from build123d import *

# Parameters (mm, degrees)
EXTRUDE_1_DEPTH                 = 52
CUT_EXTRUDE_1_REACH             = 161.013
CUT_EXTRUDE_1_DIRECTION_2_DEPTH = 7
SKETCH_3_R                      = 1.5
SKETCH_3_R_2                    = 3
CUT_EXTRUDE_2_DEPTH             = 160.138304628
FILLET_1_R                      = 5
CHAMFER_1_SIZE                  = 5
FILLET_2_R                      = 12.5
EXTRUDE_2_DEPTH                 = 9
EXTRUDE_3_DEPTH                 = 9
EXTRUDE_3_DEPTH_BACK            = 2
CHAMFER_3_SIZE                  = 6
EXTRUDE_START                   = -11
SKETCH_7_R                      = 1.6
EXTRUDE_4_DEPTH                 = 2


with BuildPart() as part:
    # 草图1 → 凸台-拉伸1 (new body)
    with BuildSketch(Plane(origin=(0, 0, 0), x_dir=(0, 0, -1), z_dir=(1, 0, 0))):
        Polygon((0, 0), (0, 98), (-9, 98), (-9, 150), (-7, 150), (-7, 100), (2, 100), (2, 0), align=None)
    extrude(amount=EXTRUDE_1_DEPTH)

    # 草图2 → 切除-拉伸1 (cut, up to next)
    with BuildSketch(Plane(origin=(0, 0, 7), x_dir=(-1, 0, 0), z_dir=(0, 0, -1)), mode=Mode.PRIVATE) as cut_extrude_1_sk1:
        Polygon((-49, 146), (-49, 123), (-24, 123), (-24, 128.5), (-14, 128.5), (-14, 117), (-41, 117), (-41, 106), (-31, 106), (-31, 98), (-17, 98), (-17, 106), (-4, 106), (-4, 140.5), (-24, 140.5), (-24, 146), align=None)
    cut_extrude_1_tool1 = extrude(cut_extrude_1_sk1.sketch, amount=-CUT_EXTRUDE_1_REACH, mode=Mode.PRIVATE) & part.part
    add(cut_extrude_1_tool1.solids().sort_by_distance((25.692202, 124.595066, 7))[0], mode=Mode.SUBTRACT)

    # 草图2 → 切除-拉伸1 direction 2 (cut)
    with BuildSketch(Plane(origin=(0, 0, 7), x_dir=(-1, 0, 0), z_dir=(0, 0, -1))):
        Polygon((-49, 146), (-49, 123), (-24, 123), (-24, 128.5), (-14, 128.5), (-14, 117), (-41, 117), (-41, 106), (-31, 106), (-31, 98), (-17, 98), (-17, 106), (-4, 106), (-4, 140.5), (-24, 140.5), (-24, 146), align=None)
    extrude(amount=CUT_EXTRUDE_1_DIRECTION_2_DEPTH, mode=Mode.SUBTRACT)

    # 草图3 → 切除-拉伸2 (cut, through all)
    with BuildSketch(Plane(origin=(0, 0, -2), x_dir=(-1, 0, 0), z_dir=(0, 0, -1))):
        with Locations(Location((-15.5, 19, 0), (0, 0, 90))):
            Circle(SKETCH_3_R)
        with Locations(Location((-12, 19, 0), (0, 0, 90))):
            Circle(SKETCH_3_R)
        with Locations(Location((-8.5, 19, 0), (0, 0, 90))):
            Circle(SKETCH_3_R)
        with Locations(Location((-8.5, 5, 0), (0, 0, 90))):
            Circle(SKETCH_3_R)
        with Locations(Location((-12, 5, 0), (0, 0, 90))):
            Circle(SKETCH_3_R)
        with Locations(Location((-15.5, 5, 0), (0, 0, 90))):
            Circle(SKETCH_3_R)
        with Locations(Location((-5, 15.5, 0), (0, 0, 90))):
            Circle(SKETCH_3_R)
        with Locations(Location((-5, 12, 0), (0, 0, 90))):
            Circle(SKETCH_3_R)
        with Locations(Location((-5, 8.5, 0), (0, 0, 90))):
            Circle(SKETCH_3_R)
        with Locations(Location((-19, 8.5, 0), (0, 0, 90))):
            Circle(SKETCH_3_R)
        with Locations(Location((-19, 12, 0), (0, 0, 90))):
            Circle(SKETCH_3_R)
        with Locations(Location((-19, 15.5, 0), (0, 0, 90))):
            Circle(SKETCH_3_R)
        with Locations(Location((-8, 145, 0), (0, 0, 90))):
            Circle(SKETCH_3_R)
        with Locations(Location((-47, 116, 0), (0, 0, 90))):
            Circle(SKETCH_3_R)
        with Locations(Location((-18, 145, 0), (0, 0, 90))):
            Circle(SKETCH_3_R)
        with Locations(Location((-12, 12, 0), (0, 0, 90))):
            Circle(SKETCH_3_R_2)
        Polygon((-42, 75), (-22, 0), (-52, 0), (-52, 115), (-42, 100), align=None)
        with BuildLine():
            Line((0, 100), (-10.111173925, 100))
            ThreePointArc((-10.111173925, 100), (-23.988643866, 58.568340451), (0, 22.048324701))
            Line((0, 22.048324701), (0, 100))
        make_face()
    extrude(amount=-CUT_EXTRUDE_2_DEPTH, mode=Mode.SUBTRACT)

    # 圆角1
    fillet_1_edges = [part.edges().sort_by_distance(p)[0] for p in [
        (0, 100, 8),
        (52, 115, 8),
        (52, 150, 8),
        (14, 128.5, 8),
        (14, 117, 8),
        (4, 106, 8),
        (4, 140.5, 8),
        (0, 150, 8),
    ]]
    fillet(fillet_1_edges, radius=FILLET_1_R)

    # 倒角1
    chamfer_1_edges = [part.edges().sort_by_distance(p)[0] for p in [
        (36.5, 100, 7),
        (13.555586963, 100, 7),
    ]]
    chamfer(chamfer_1_edges, length=CHAMFER_1_SIZE)

    # 圆角2
    # the kernel refuses this fillet: 12.5 mm, written as the material it takes off along each edge
    with BuildSketch(Plane(origin=(22, 0, -26.008697284), x_dir=(0.2576626505603326, 0.9662349396012463, 0), z_dir=(0, 0, 1))) as fillet_2_piece_1:
        with BuildLine():
            CenterArc((FILLET_2_R * 0.768278313084, FILLET_2_R), FILLET_2_R, 194.931417178, 75.068582822)
            Line((-FILLET_2_R * 0.197956626517, FILLET_2_R * 0.74233734944), (0, 0))
            Line((0, 0), (FILLET_2_R * 0.768278313084, 0))
        make_face()
    extrude(amount=50.017394568, mode=Mode.SUBTRACT)
    with BuildSketch(Plane(origin=(0, 0, -33.25), x_dir=(1, 0, 0), z_dir=(0, 0, 1))) as fillet_2_piece_2:
        with BuildLine():
            CenterArc((FILLET_2_R, FILLET_2_R), FILLET_2_R, 180, 90)
            Line((0, FILLET_2_R), (0, 0))
            Line((0, 0), (FILLET_2_R, 0))
        make_face()
    extrude(amount=64.5, mode=Mode.SUBTRACT)
    with BuildSketch(Plane(origin=(0, 22.048324701, -18.489371261), x_dir=(0.8273370938030895, 0.561705735432226, 0), z_dir=(0, 0, 1))) as fillet_2_piece_3:
        with BuildLine():
            CenterArc((6.636843908, -12.478229092), FILLET_2_R, 93.382080567, 52.444076451)
            Line((-3.704869764, -5.456907399), (0, 0))
            ThreePointArc((0, 0), (2.949708404, -0.087083632), (5.899416807, 0))
        make_face()
    extrude(amount=34.978742522, mode=Mode.SUBTRACT)

    # 草图4 → 凸台-拉伸2 (add)
    with BuildSketch(Plane(origin=(0, 0, 7), x_dir=(-1, 0, 0), z_dir=(0, 0, -1))):
        Polygon((-24, 128.5), (-24, 123), (-49, 123), (-49, 146), (-24, 146), (-24, 140.5), (-22.5, 140.5), (-22.5, 147.5), (-50.5, 147.5), (-50.5, 121.5), (-45, 121.5), (-42, 100), (-40.485467906, 100), (-43.485467906, 121.5), (-22.5, 121.5), (-22.5, 128.5), align=None)
    extrude(amount=EXTRUDE_2_DEPTH)

    # 草图6 → 凸台-拉伸3 (add, two sides: drawn at the far end of the back side and taken through both)
    with BuildSketch(Plane.XY.offset(-EXTRUDE_3_DEPTH_BACK)):
        with BuildLine():
            Line((42, 98), (42, 75))
            Line((42, 75), (24.474457831, 9.279216868))
            ThreePointArc((24.474457831, 9.279216868), (10.631728691, -0.694195235), (-0.76772333, 12))
            Line((-0.76772333, 12), (0.709641329, 12))
            ThreePointArc((0.709641329, 12), (10.981525419, 0.755672166), (23.10661066, 9.971355488))
            Line((23.10661066, 9.971355488), (40.5, 75.196565511))
            Line((40.5, 75.196565511), (40.5, 98))
            Line((40.5, 98), (42, 98))
        make_face()
    extrude(amount=EXTRUDE_3_DEPTH + EXTRUDE_3_DEPTH_BACK)

    # 倒角3
    chamfer_3_edges = [part.edges().sort_by_distance(p)[0] for p in [
        (14.483655862, 98, 0),
        (35.75, 98, 0),
    ]]
    chamfer(chamfer_3_edges, length=CHAMFER_3_SIZE)

    # 草图7 → 凸台-拉伸4 (add)
    with BuildSketch(Plane(origin=(0, 0, -2), x_dir=(-1, 0, 0), z_dir=(0, 0, -1)).offset(EXTRUDE_START)):
        with BuildLine():
            Line((-39.167379443, 64.377672911), (-42.901819277, 63.381822289))
            ThreePointArc((-42.901819277, 63.381822289), (-45.381822289, 59.098180723), (-41.098180723, 56.618177711))
            Line((-41.098180723, 56.618177711), (-37.363740889, 57.614028334))
            Line((-37.363740889, 57.614028334), (-39.167379443, 64.377672911))
        make_face()
        with Locations(Location((-42, 60, 0), (0, 0, 90))):
            Circle(SKETCH_7_R, mode=Mode.SUBTRACT)
    extrude(amount=EXTRUDE_4_DEPTH)


solid = part.part
Check sheet for the modelled part. Datum: model origin and axes. Units: mm. A direction names the side the tool comes from. Round coordinates to 2 decimals unless told otherwise and drop trailing zeros. Loops run counter-clockwise (first coordinate to the right, second up) from the corner with the lowest first, then second, coordinate; pieces in that order, holes last. Notation, with made-up numbers: M -17,-9 L -2,-9 A23 cw -2,2 Z; hole C 77.5,-20.5 d1. An arc over 180 degrees is marked long. One line per item, written item: value.
(1) Release check for a two-part mould opening along X. For faces 6 (the face through (43, 103, 5)), 7 (the face through (23, 128.5, 5)), 8 (the face through (1, 148, 8)) record: +X half, -X half, draft (parallel to the pull), parting line (faces both ways), or undercut.
Computed values:
face 6: draft
face 7: undercut
face 8: -X half
(2) Depth check by flat-ended pin: pin 1 Ø4.5 at (y, z) = (84.5, 3.5) entering from -X; pin 2 Ø8 at (x, y) = (19, 44.5) entering from +Z; pin 3 Ø3 at (y, z) = (53, 3.5) entering from +X. Enter the tip coordinate at first touch or a pass-through.
Computed values:
pin 1: stops at x = 40.5
pin 2: stops at z = 0
pin 3: stops at x = 36.53
(3) Sectioned sample at D-D, the plane x = 35. Record the cut outline in (y, z).
Computed values:
outline: M 48.75,-2 L 100,-2 L 100,2 L 105,7 L 106,7 L 106,9 L 98,9 L 98,6 L 92,0 L 54.57,0 L 54.57,9 L 48.75,9 Z; M 117,7 L 121.5,7 L 121.5,-2 L 123,-2 L 123,9 L 117,9 Z; M 146,-2 L 147.5,-2 L 147.5,7 L 150,7 L 150,9 L 146,9 Z
(4) Thickness scan on line 1 (X direction, y = 145, z = 7.8); line 2 (X direction, y = 116, z = 7.85); line 3 (X direction, y = 95.5, z = 2). Record the ranges inside material, lowest first.
Computed values:
line 1: x = 0 to 6.5, 9.5 to 16.5, 19.5 to 24, 49 to 52
line 2: x = 0 to 4, 41 to 45.5, 48.5 to 51.97
line 3: x = 14.02 to 17, 31 to 42
(5) Sectioned sample at A-A, the plane y = 119.5. Record the cut outline in (x, z).
Computed values:
outline: M 0,7 L 4,7 L 4,9 L 0,9 Z; M 14.67,7 L 43.21,7 L 43.21,-2 L 44.72,-2 L 44.72,7 L 52,7 L 52,9 L 14.67,9 Z
(6) Access from +Z, -Z, +X, -X, +Y, -Y to the whole of each face (thin tool, end or side, straight path). Record for faces 1 (the face through (36, 147.5, 3)), 2 (the face through (24, 143, 4)), 3 (the face through (10.75, 0.78, 4.44)), 4 (the face through (22.5, 144, 3)), 5 (the face through (40.6, 61.4, 7)).
Computed values:
face 1: -Z, +X, -X, +Y
face 2: +Z, -Z
face 3: +Z
face 4: -Z, -X, +Y
face 5: -Z, +X, -Y
(7) Sectioned sample at C-C, the plane y = 19. Record the cut outline in (x, z), then the cut area to 3 significant figures.
Computed values:
outline: M 0.51,-2 L 7,-2 L 7,0 L 0.51,0 Z; M 10,-2 L 10.5,-2 L 10.5,0 L 10,0 Z; M 13.5,-2 L 14,-2 L 14,0 L 13.5,0 Z; M 17,-2 L 27.07,-2 L 27.07,9 L 25.51,9 L 25.51,0 L 17,0 Z
area: 49.1 mm^2
